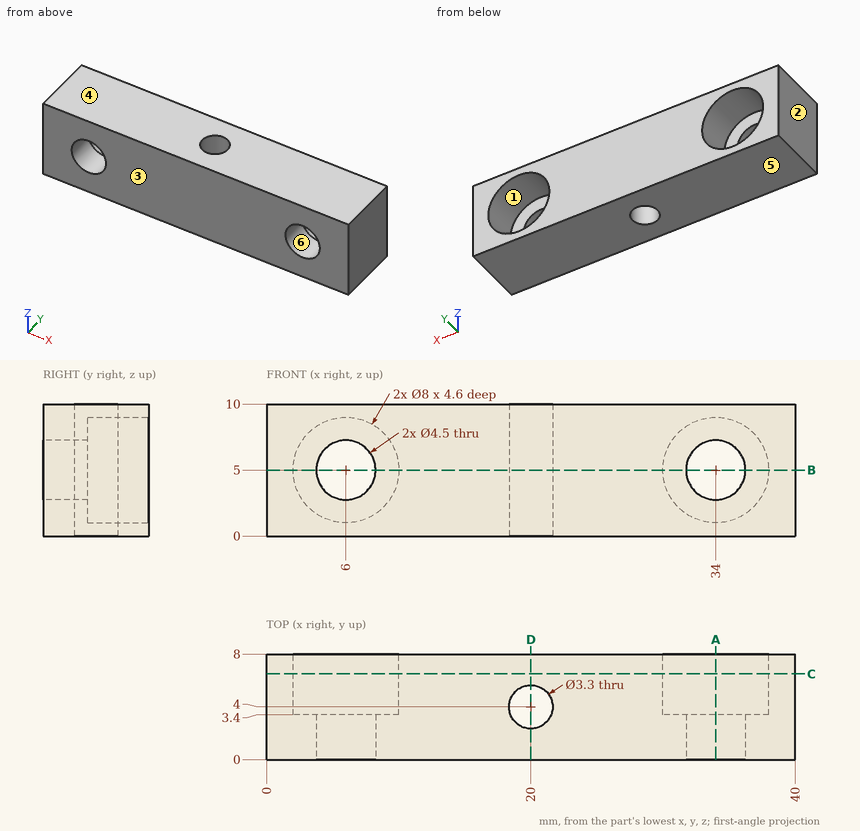
Geometry: see drawing. Coordinates: mm, zero at the bounding-box minimum. A direction names the side the tool comes from. Round coordinates to 2 decimals unless told otherwise and drop trailing zeros. Write each loop counter-clockwise with the first axis right and the second up, starting at its lowest first coordinate (ties: lowest second). Pieces come first, ordered by that corner, then holes.
1) Draft query along Z for the marked faces 3, 4, 5 and 6. Return one class per face: pulls with the +Z half, pulls with the -Z half, needs draft (parallel to the pull), parting line crosses it, or undercut.
2) Ray query, L1, parallel to Z at x = 34, y = 2.45; L2, parallel to Z at x = 6, y = 4.5; L3, parallel to X at y = 1.5, z = 3. Return the intervals inside material, ascending.
3) Cut plane C-C (y = 6.5). Return the cut outline in (x, z).
4) Cut plane D-D (x = 20). Return the cut outline in (y, z).
5) Cut plane B-B (z = 5). Return the cut outline in (x, y).
6) Cut plane A-A (x = 34). Return the cut outline in (y, z).
7) Reachability of the marked faces 1 and 2 from +Z, -Z, +X, -X, +Y, -Y: full face, straight path, thin tool, end or side. Return the list, or none.
Geometry says:
1. face 3: needs draft
1. face 4: pulls with the +Z half
1. face 5: pulls with the -Z half
1. face 6: undercut
2. L1: z = 0 to 2.75, 7.25 to 10
2. L2: z = 0 to 1, 9 to 10
2. L3: x = 0 to 4.97, 7.03 to 32.97, 35.03 to 40
3. outline: (0, 0) - (40, 0) - (40, 10) - (0, 10) - close; hole circle Ø8 at (6, 5); hole circle Ø8 at (34, 5)
4. outline: (0, 0) - (2.35, 0) - (2.35, 10) - (0, 10) - close; (5.65, 0) - (8, 0) - (8, 10) - (5.65, 10) - close
5. outline: (0, 0) - (3.75, 0) - (3.75, 3.4) - (2, 3.4) - (2, 8) - (0, 8) - close; (8.25, 0) - (31.75, 0) - (31.75, 3.4) - (30, 3.4) - (30, 8) - (10, 8) - (10, 3.4) - (8.25, 3.4) - close; (36.25, 0) - (40, 0) - (40, 8) - (38, 8) - (38, 3.4) - (36.25, 3.4) - close; hole circle Ø3.3 at (20, 4)
6. outline: (0, 0) - (8, 0) - (8, 1) - (3.4, 1) - (3.4, 2.75) - (0, 2.75) - close; (0, 7.25) - (3.4, 7.25) - (3.4, 9) - (8, 9) - (8, 10) - (0, 10) - close
7. face 1: +Y
7. face 2: +Z, -Z, -X, +Y, -Y
